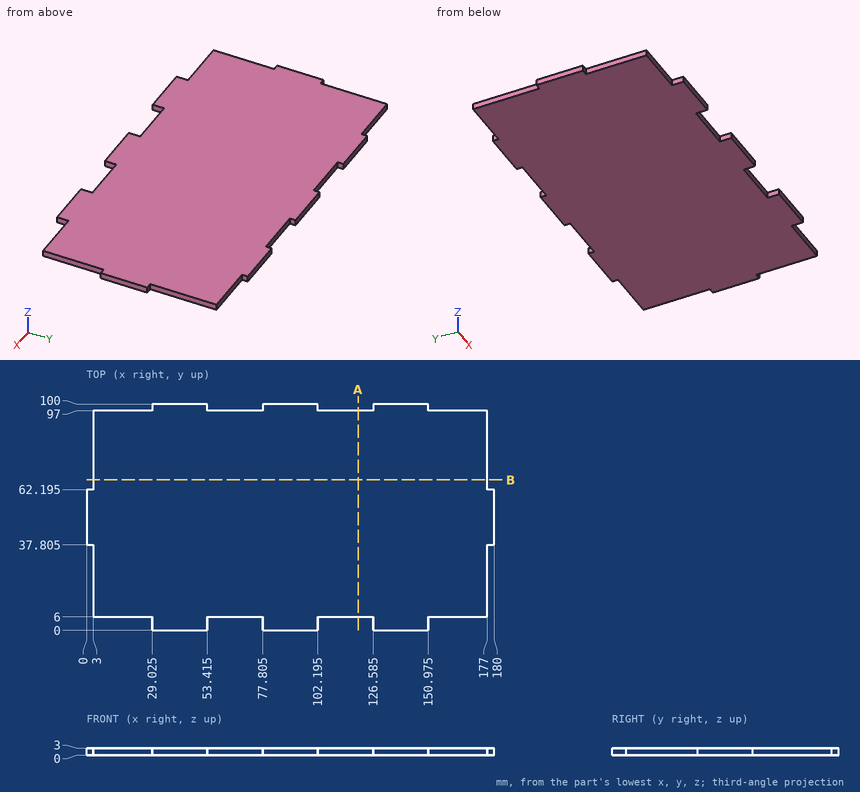
Design review of the part shown in the three views and the two pictorial views. Dimensions are in mm from the part's minimum x, y and z. Round coordinates to 2 decimals unless told otherwise and drop trailing zeros. Loops run counter-clockwise (first coordinate to the right, second up) from the corner with the lowest first, then second, coordinate; pieces in that order, holes last. Notation, with made-up numbers: (35, 9.25) -> (46, 9.25) arc R14 cw to (46, 21.25) -> close; hole circle Ø3 at (46.5, 60). An arc over 180 degrees is marked (long way). Answer as CSV lines item,"result".
1) Add section B-B on y = 66.5. Write out the cut boundary in (x, z), plus the area to 3 significant figures.
Geometry results:
outline,"(3, 0) -> (177, 0) -> (177, 3) -> (3, 3) -> close"
area,"522 mm²"
2) For P1, Ø8, axis at x = 109.5, y = 41.5, coming from the -Z side; P2, Ø0.9, axis at x = 70.5, z = 1, coming from the +Y side; P3, Ø1.5, axis at y = 98.5, z = 2, coming from the +X side (3 decimals); P4, Ø1.5, axis at y = 98.5, z = 1, coming from the -X side (3 decimals), all flat-tipped, find the tip position at first contact; note any pin that passes through.
Geometry results:
P1,"stops at z = 0"
P2,"stops at y = 97"
P3,"stops at x = 150.975"
P4,"stops at x = 29.025"
3) To check wall thickness, follow line 1 along X through (y, z) = (5.5, 1) (3 decimals); line 2 along X through (y, z) = (27, 0.5); line 3 along Y through (x, z) = (76, 1.4). State the ranges of each line that lie inside material, in increasing order. Write a range as from..to.
Geometry results:
line 1,"x = 29.025..53.415, 77.805..102.195, 126.585..150.975"
line 2,"x = 3..177"
line 3,"y = 6..97"
4) Add section A-A on x = 120. Write out the cut boundary in (y, z), plus the area to 3 significant figures.
Geometry results:
outline,"(6, 0) -> (97, 0) -> (97, 3) -> (6, 3) -> close"
area,"273 mm²"
